Build history of the part. All positions in model axes, mm. Coordinates: 2 decimals unless noted, no trailing zeros. Order: outer loops, then holes, each group sorted by start corner. A loop starts at its lowest first (then second) coordinate and runs counter-clockwise, first axis right, second up. Notation, with made-up numbers: (-6.5, 20) - (28.5, 20) arc R11 cw to (28.5, 32) - close; hole circle Ø5 at (68, -19). An arc over 180 degrees is marked (long way). One line per item, written item: value.
Autodesk Inventor part; units mm, degrees
ref_plane "YZ Plane" through (0, 0, 0) normal (1, 0, 0) x (0, 1, 0)
ref_plane "XZ Plane" through (0, 0, 0) normal (0, 1, 0) x (-1, 0, 0)
ref_plane "XY Plane" through (0, 0, 0) normal (0, 0, 1) x (1, 0, 0)
sketch "Sketch3" plane through (0, 0, 0) normal (0, 0, 1) x (1, 0, 0)
  arc A0 (6.2115, -31.9009) -> (6.2115, 31.9009) centre (0, 0) ccw
  line L0 (6.2115, 27.4733) -> (6.2115, 31.9009)
  line L1 (6.2115, 31.9009) -> (6.2115, -31.9009)
  circle A1 centre (0, 0) radius 42.5
  line L2 (6.2115, -31.9009) -> (6.2115, -42.0436)
  line L3 (6.2115, 31.9009) -> (6.2115, 42.0436)
  point P0 (-5.2115, 24.6247)
  dimension "d14" = 85
extrude "Extrusion2" add sketch "Sketch3" along normal blind 7.5 contours L1 L0 A0
sketch "Sketch4" plane through (6.2115, -31.9009, 0) normal (-1, 0, 0) x (0, 0, 1)
  line L0 (0, 0) -> (0, 6.9167)
  line L1 (7.5, 26.7893) -> (7.5, 0)
  line L2 (7.5, 6.9167) -> (7.5, 0)
  line L3 (7.5, 0) -> (0, 0)
  line L4 (7.5, 0) -> (0, 0)
  circle A0 centre (3.75, 8.5699) radius 1
  line L5 (0, 0) -> (3.0149, 2.7804)
  line L6 (4.4851, 4.1363) -> (7.5, 6.9167)
  line L7 (0, 6.9167) -> (3.0149, 4.1363)
  line L8 (4.4851, 2.7804) -> (7.5, 0)
  line L9 (0, 0) -> (0, 53.5786)
  line L10 (0, 53.5786) -> (0, 0)
  line L11 (0, 31.9009) -> (7.5, 31.9009)
  circle A1 centre (3.75, 55.2319) radius 1
  line L12 (7.5, 53.5786) -> (7.5, 0)
  line L13 (0, 0) -> (0, 63.8018)
  line L14 (0, 63.8018) -> (0, 0)
  line L15 (0, 31.9009) -> (3.75, 31.9009)
  circle A2 centre (3.75, 8.5699) radius 2
  circle A3 centre (3.75, 55.2319) radius 2
  point P0 (280.32, 51.414)
  dimension "d7" = 2
  dimension "d10" = 4
  dimension "d11" = 4
extrude "Extrusion3" cut sketch "Sketch4" against normal blind 25.4 contours A0 | A1
extrude "Extrusion4" cut sketch "Sketch4" against normal blind 32.8625 contours A2 | A3
extrude "Extrusion5" add sketch "Sketch3" along normal blind 7.5 contours A0 L3 A1 L2
extrude "Extrusion6" cut sketch "Sketch4" against normal blind 50.3625 contours A0 | A1 | A2 | A3
scale "Scale1" factors (0.5, 0.5, 0.5) then translate (3.1057, 0, 0) bodies 1
properties part number "ContrapesoGrande"
1. Band-saw the part on C-C, the plane y = 4. Give the cut face in (x, z), and give its area (3 significant figures).
Values found:
outline: (6.21, 0) - (23.98, 0) - (23.98, 3.75) - (6.21, 3.75) - close
area: 66.6 mm2
2. Probe line 1 along Y through (x, z) = (17, 2.55); line 2 along Y through (x, z) = (7, 1.95); line 3 along X through (y, z) = (0, 1.25). List the from-to ranges inside material, lowest first.
Values found:
line 1: y = -16.08 to -12.4, -10.93 to 10.93, 12.4 to 16.08
line 2: y = -20.89 to -12.66, -10.67 to 10.67, 12.66 to 20.89
line 3: x = 6.21 to 24.36
3. Band-saw the part on A-A, the plane z = 2.1. Give the cut face in (x, y), and give its area (3 significant figures).
Values found:
outline: (6.21, -21.02) arc R21.25 ccw to (20.19, -12.64) - (6.21, -12.64) - close; (6.21, -10.69) - (21.47, -10.69) arc R21.25 ccw to (21.47, 10.69) - (6.21, 10.69) - close; (6.21, 12.64) - (20.19, 12.64) arc R21.25 ccw to (6.21, 21.02) - close
area: 521 mm2
4. Two-plate mould, pull along Y, no slides. Class faces 1 (the face through (13.742, -10.674, 1.745)), 2 (the face through (24.35, 0.42, 1.85)), 3 (the face through (6.211, 0, 2)): pulls with the +Y half, pulls with the -Y half, needs draft (parallel to the pull), parting line crosses it, or undercut.
Values found:
face 1: undercut
face 2: parting line crosses it
face 3: needs draft
5. Band-saw the part on B-B, the plane x = 10.25. Count the separate pieces of the cut face and the enclosed holes in it, and give its area (3 significant figures).
Values found:
separate pieces: 1
enclosed holes: 2
area: 144 mm2
6. Flat gauge pins, fed straight in: P1, Ø1.2, axis at y = -11.67, z = 1.88, coming from the -X side; P2, Ø1, axis at y = -8.5, z = 1, coming from the +X side. Where does each tip first touch, or does it go through?
Values found:
P1: passes through
P2: stops at x = 22.79
